from build123d import *

# Parameters (mm, degrees)
F1_DEPTH = 6.35
F2_W     = 6.35
F2_H     = 50.8
F3_DEPTH = 673.1
F5_DEPTH = 6.35
F6_W     = 50.8
F6_H     = 6.35
F7_DEPTH = 673.1


with BuildPart() as f1:
    # F0 (on Top) → F1 (new body)
    with BuildSketch(Plane.XY):
        Polygon((457.2, 0), (0, 0), (0, 457.2), (-50.8, 457.2), (-50.8, -50.8), (457.2, -50.8), align=None)
    extrude(amount=F1_DEPTH)

    # F2 (on face) → F3 (join)
    with BuildSketch(Plane(origin=(0, 0, 0), x_dir=(1, 0, 0), z_dir=(0, 0, -1))):
        with Locations((454.025, 25.4)):
            Rectangle(F2_W, F2_H)
    extrude(amount=F3_DEPTH)

    # F4 (on face) → F5 (join)
    with BuildSketch(Plane(origin=(0, 0, -673.1), x_dir=(1, 0, 0), z_dir=(0, 0, -1))):
        Polygon((457.2, 0), (457.2, 50.8), (-50.8, 50.8), (-50.8, -457.2), (0, -457.2), (0, 0), align=None)
    extrude(amount=F5_DEPTH)

    # F6 (on face) → F7 (join, through all)
    with BuildSketch(Plane(origin=(0, 0, 0), x_dir=(1, 0, 0), z_dir=(0, 0, -1))):
        with Locations((-25.4, -454.025)):
            Rectangle(F6_W, F6_H)
    extrude(amount=F7_DEPTH)


solid = f1.part
Build history of the part. All positions in model axes, mm. A direction names the side the tool comes from. Give positions to 0.01 mm unless a question says otherwise; leave off trailing zeros. Write each loop counter-clockwise with the first axis right and the second up, starting at its lowest first coordinate (ties: lowest second). Pieces come first, ordered by that corner, then holes. Notation, with made-up numbers: (-19, 43.5) - (1, 43.5) arc R18 cw to (1, 51.5) - close; hole circle Ø7 at (83, 14). An arc over 180 degrees is marked (long way). Use one line per item in the form item = value. Start each with the question number.
1. Two-plate mould, pull along Z, no slides. Class faces 3 (the face through (450.85, -25, -332)), 4 (the face through (89, -3, 6.35)), 5 (the face through (-26, 450.85, -332)), 6 (the face through (-5, 89, -679.45)): released by +Z, released by -Z, zero draft, split by the parting line, or undercut.
2. 3-axis set-ups, long thin cutter, end or side, ignore diameter. For faces 1 (the face through (-6, 87, -673.1)), 2 (the face through (-26, 457.2, -332)): which of +Z, -Z, +X, -X, +Y, -Y reach the whole face in a straight line?
3. Band-saw the part on A-A on y = 409.5. Write the cut outline in (x, z).
4. Probe line 1 (Z direction, x = -27.5, y = 100.5); line 2 (Y direction, x = -27, z = -363.5). List the from-to ranges inside material, lowest first. Write a range as [from, to].
5. Drop a flat-ended pin along its axis: pin 1 Ø15 at (y, z) = (-26.5, -332.5) entering from -X. Give the stop position or say it passes through.
Conclusion:
q1.face_3 = undercut
q1.face_4 = released by +Z
q1.face_5 = undercut
q1.face_6 = released by -Z
q2.face_1 = -X, -Y
q2.face_2 = +Z, -Z, +X, -X, +Y
q3.outline = (-50.8, -679.45) - (0, -679.45) - (0, -673.1) - (-50.8, -673.1) - close; (-50.8, 0) - (0, 0) - (0, 6.35) - (-50.8, 6.35) - close
q4.line_1 = [-679.45, -673.1], [0, 6.35]
q4.line_2 = [450.85, 457.2]
q5.pin_1 = 450.85
